from build123d import *

# Parameters (mm, degrees)
EXTRUDE_1_DEPTH = 3
CHAMFER_1_SIZE  = 0.2


with BuildPart() as part:
    # 草图1 → 旋转2 (revolve)
    with BuildSketch(Plane.XY, mode=Mode.PRIVATE) as revolve_2_sk:
        with BuildLine():
            Line((-1, 18), (-2.4, 18))
            Line((-2.4, 18), (-3.3, 16.271116086))
            Line((-3.3, 16.271116086), (-2.8, 14.675583457))
            ThreePointArc((-2.8, 14.675583457), (-3.219653878, 12.154380629), (-5.5, 11))
            Line((-5.5, 11), (-5.5, 8))
            Line((-5.5, 8), (-5, 8))
            Line((-5, 8), (-5, 3.643969354))
            Line((-5, 3.643969354), (-1.5, 1.821984677))
            Line((-1.5, 1.821984677), (-1.5, 0))
            Line((-1.5, 0), (-1, 0))
            Line((-1, 0), (-1, 18))
        make_face()
    revolve(revolve_2_sk.sketch.rotate(Axis((0, 0, 0), (0, -1, 0)), 270), axis=Axis((0, 0, 0), (0, -1, 0)))

    # 草图2 → 拉伸1 (add)
    with BuildSketch(Plane.XZ.offset(-8)):
        Polygon((-5.5, 3.175426481), (-5.5, -3.175426481), (0, -6.350852961), (5.5, -3.175426481), (5.5, 3.175426481), (0, 6.350852961), align=None)
    extrude(amount=-EXTRUDE_1_DEPTH)

    # 倒角1
    chamfer_1_edges = [part.edges().sort_by_distance(p)[0] for p in [
        (0, 0, -1.5),
    ]]
    chamfer(chamfer_1_edges, length=CHAMFER_1_SIZE)


solid = part.part
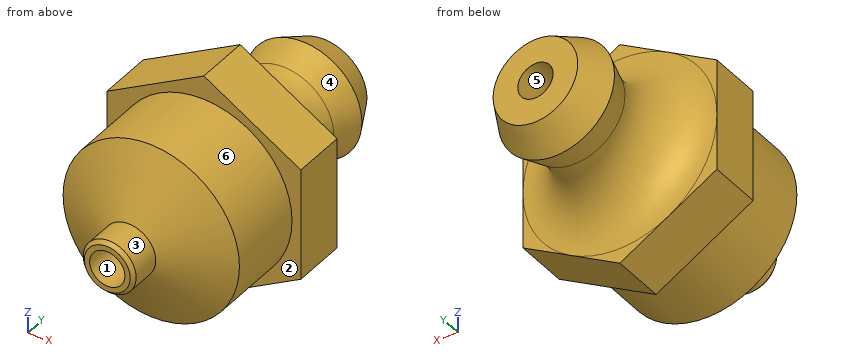
Part model, mm, in its own coordinate system. Face numbers are marked on the shaded views. A direction names the side the tool comes from. Coordinates: 2 decimals unless noted, no trailing zeros. Write each loop counter-clockwise with the first axis right and the second up, starting at its lowest first coordinate (ties: lowest second). Pieces come first, ordered by that corner, then holes. Notation, with made-up numbers: M 61,85 L 92,85 A20 ccw 92,92 Z; hole C 63,13 d11. An arc over 180 degrees is marked long. Return JSON: item names as keys, results as strings.
1. Saw through at B-B, the plane y = 12.25. Write the cut outline in (x, z), then the cut area to 3 significant figures.
Determined:
{"outline": "C 0,0 d6.3; hole C 0,0 d2", "area": "28.1 mm²"}
2. 3-axis set-ups, long thin cutter, end or side, ignore diameter. For the marked faces 4, 5 and 6: which of +Z, -Z, +X, -X, +Y, -Y reach the whole face in a straight line?
Determined:
{"face 4": "none", "face 5": "+Y", "face 6": "-Y"}
3. Flat gauge pins, fed straight in: pin 1 Ø3 at (x, z) = (4, 2.5) entering from +Y; pin 2 Ø3 at (x, z) = (0, 0) entering from -Y; pin 3 Ø2 at (y, z) = (5.5, -0.5) entering from -X; pin 4 Ø2 at (x, y) = (0, 12.5) entering from +Z. Where does each tip first touch, or does it go through?
Determined:
{"pin 1": "y = 16.43", "pin 2": "y = 0", "pin 3": "x = -5", "pin 4": "z = 3.89"}
4. Saw through at A-A, the plane y = 10. Write the cut outline in (x, z).
Determined:
{"outline": "M -5.5,-3.18 L 0,-6.35 L 5.5,-3.18 L 5.5,3.18 L 0,6.35 L -5.5,3.18 Z"}
5. Saw through at C-C, the plane z = 5.75. Write the cut outline in (x, y), then the cut area to 3 significant figures.
Determined:
{"outline": "M -1.04,8 L 1.04,8 L 1.04,11 L -1.04,11 Z", "area": "6.24 mm²"}
6. Pull direction Z, two halves, no side cores. Call the marked faces 1, 2 and 3: pulls with the +Z half, pulls with the -Z half, needs draft (parallel to the pull), parting line crosses it, or undercut.
Determined:
{"face 1": "undercut", "face 2": "needs draft", "face 3": "parting line crosses it"}
7. Probe L1, parallel to X at y = 1, z = 0; L2, parallel to Y at x = -3.75, z = 4; L3, parallel to X at y = 12.5, z = 0. List the from-to ranges inside material, lowest first.
Determined:
{"L1": "-1.5 to -1, 1 to 1.5", "L2": "8 to 11", "L3": "-3 to -1, 1 to 3"}
